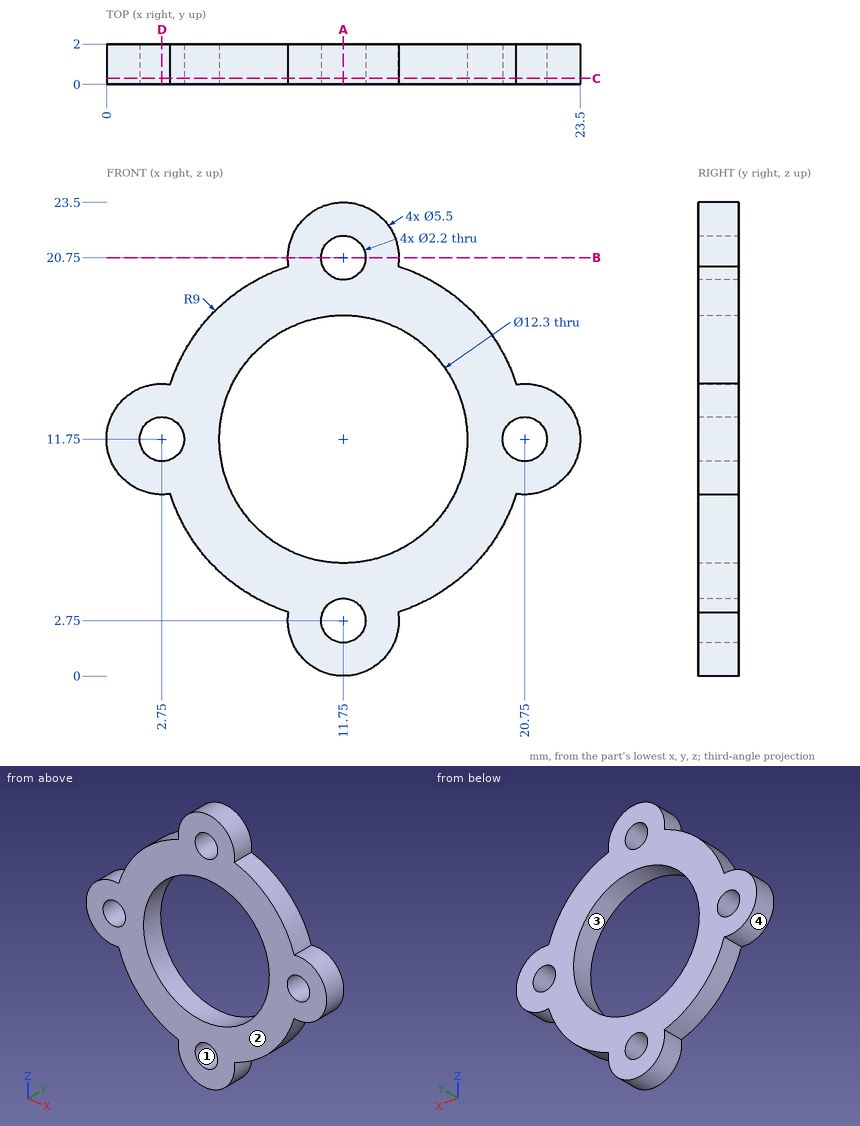
Job drawing, mm, ordinate dimensions from the low corner. One solid piece. Round coordinates to 2 decimals unless told otherwise and drop trailing zeros. Write each loop counter-clockwise with the first axis right and the second up, starting at its lowest first coordinate (ties: lowest second). Pieces come first, ordered by that corner, then holes. Notation, with made-up numbers: (81.25, 6) -> (119.25, 6) arc R23 ccw to (119.25, 17) -> close; hole circle Ø10 at (88, 26). An arc over 180 degrees is marked (long way). Answer as a JSON object with one key per item and string values.
(1) Band-saw the part on B-B, the plane z = 20.75. List the corners of the cut face in (x, y), then the cut area to 3 significant figures.
Reported:
{"outline": "(9, 0) -> (10.65, 0) -> (10.65, 2) -> (9, 2) -> close; (12.85, 0) -> (14.5, 0) -> (14.5, 2) -> (12.85, 2) -> close", "area": "6.60 mm^2"}
(2) Two-plate mould, pull along Z, no slides. Class the marked faces 1, 2, 3 and 4: +Z half, -Z half, draft (parallel to the pull), parting line (faces both ways), or undercut.
Reported:
{"face 1": "undercut", "face 2": "draft", "face 3": "undercut", "face 4": "parting line"}
(3) Band-saw the part on C-C, the plane y = 0.3. List the corners of the cut face in (x, z), then the cut area to 3 significant figures.
Reported:
{"outline": "(3.17, 9.03) arc R9 ccw to (9.03, 3.17) arc R2.75 ccw (long way) to (14.47, 3.17) arc R9 ccw to (20.33, 9.03) arc R2.75 ccw (long way) to (20.33, 14.47) arc R9 ccw to (14.47, 20.33) arc R2.75 ccw (long way) to (9.03, 20.33) arc R9 ccw to (3.17, 14.47) arc R2.75 ccw (long way) to start; hole circle Ø2.2 at (2.75, 11.75); hole circle Ø12.3 at (11.75, 11.75); hole circle Ø2.2 at (11.75, 2.75); hole circle Ø2.2 at (11.75, 20.75); hole circle Ø2.2 at (20.75, 11.75)", "area": "171 mm^2"}
(4) Band-saw the part on A-A, the plane x = 11.75. List the corners of the cut face in (y, z).
Reported:
{"outline": "(0, 0) -> (2, 0) -> (2, 1.65) -> (0, 1.65) -> close; (0, 3.85) -> (2, 3.85) -> (2, 5.6) -> (0, 5.6) -> close; (0, 17.9) -> (2, 17.9) -> (2, 19.65) -> (0, 19.65) -> close; (0, 21.85) -> (2, 21.85) -> (2, 23.5) -> (0, 23.5) -> close"}
(5) Band-saw the part on D-D, the plane x = 2.75. List the corners of the cut face in (y, z), then the cut area to 3 significant figures.
Reported:
{"outline": "(0, 9) -> (2, 9) -> (2, 10.65) -> (0, 10.65) -> close; (0, 12.85) -> (2, 12.85) -> (2, 14.5) -> (0, 14.5) -> close", "area": "6.60 mm^2"}
(6) Probe probe 1 along X at (y, z) = (0.9, 11.75); probe 2 along X at (y, z) = (1.15, 12.75); probe 3 along X at (y, z) = (1.2, 13). List the from-to ranges inside material, lowest first. Write a range as [from, to].
Reported:
{"probe 1": "x = [0, 1.65], [3.85, 5.6], [17.9, 19.65], [21.85, 23.5]", "probe 2": "x = [0.19, 2.29], [3.21, 5.68], [17.82, 20.29], [21.21, 23.31]", "probe 3": "x = [0.3, 5.73], [17.77, 23.2]"}
